Here's the drawing with two shaded views (mm, measured from the low corner). I have some questions. A direction names the side the tool comes from. Give positions to 0.01 mm unless a question says otherwise; leave off trailing zeros. Loops run counter-clockwise (first coordinate to the right, second up) from the corner with the lowest first, then second, coordinate; pieces in that order, holes last. Notation, with made-up numbers: (89.5, 50) - (136.5, 50) arc R12 cw to (136.5, 63) - close; hole circle Ø8 at (86.5, -29). An arc over 180 degrees is marked (long way). Answer as a JSON object with one key per item and string values. Group by question number.
Item 1: Suppose I cut it at B-B on y = 4.5. Write out the boundary of the cut face in (x, z), and give its area (3 significant figures).
Item 2: Will this pin go through, and if not, where does the flat tip stop? pin 1 (4 mm diameter, centred on x = 6.78, y = 6.73, fed in from -Z).
Item 3: Suppose I cut it at A-A on x = 30. Write out the boundary of the cut face in (y, z).
Item 4: Suppose I cut it at C-C on z = 4.75. Count the separate pieces of the cut face and the enclosed holes in it, and give its area (3 significant figures).
Item 5: Please list where these lines run through material, in increasing order: L1, parallel to Y at x = 19, z = 3.25; L2, parallel to Y at x = 30, z = 3.75; L3, parallel to X at y = 10, z = 2.75.
Item 6: Which directions (+Z, -Z, +X, -X, +Y, -Y) give clear straight access to the entire face, cutting with the end or side of a thin tool? Please do the marked faces 4 and 5.
Item 7: Thinking about a two-plate mould opening in X: for the marked faces 1, 2 and 3, which applies, pulls with the +X half, pulls with the -X half, needs draft (parallel to the pull), parting line crosses it, or undercut?
Item 8: Suppose I cut it at D-D on x = 19. Write out the boundary of the cut face in (y, z).
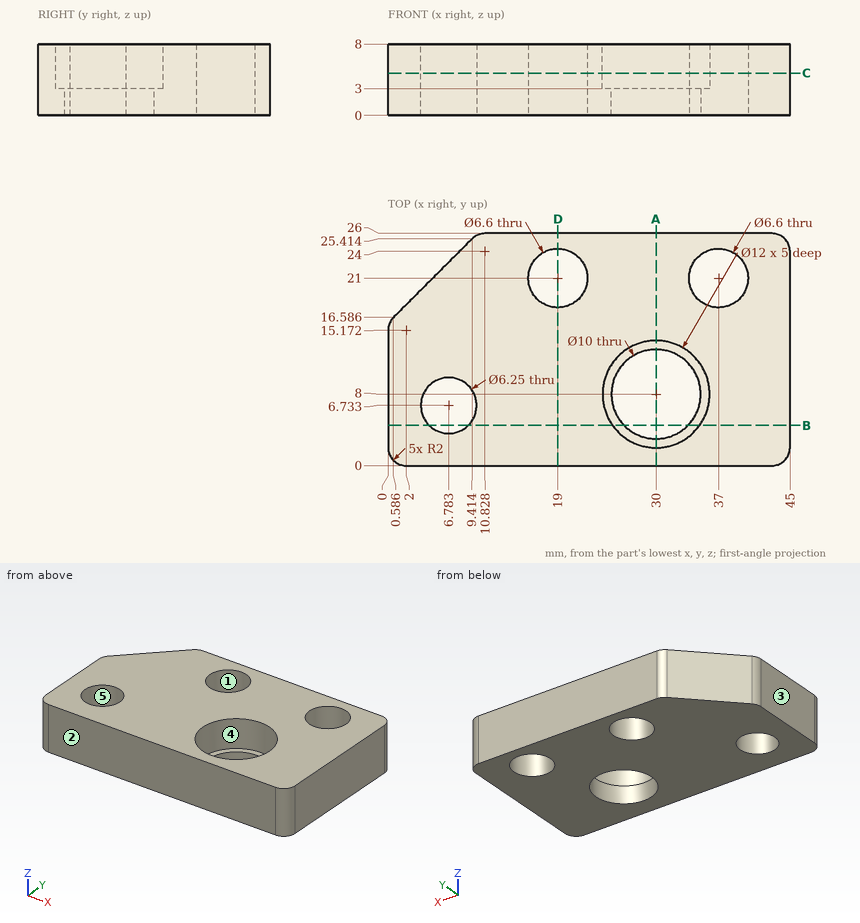
Worked out:
{
 "1": {"outline": "(0, 0) - (4.6, 0) - (4.6, 8) - (0, 8) - close; (8.97, 0) - (26.43, 0) - (26.43, 3) - (25.13, 3) - (25.13, 8) - (8.97, 8) - close; (33.57, 0) - (45, 0) - (45, 8) - (34.87, 8) - (34.87, 3) - (33.57, 3) - close", "area": "255 mm2"},
 "2": {"pin 1": "passes through"},
 "3": {"outline": "(0, 0) - (3, 0) - (3, 3) - (2, 3) - (2, 8) - (0, 8) - close; (13, 0) - (26, 0) - (26, 8) - (14, 8) - (14, 3) - (13, 3) - close"},
 "4": {"separate pieces": "1", "enclosed holes": "4", "area": "905 mm2"},
 "5": {"L1": "y = 0 to 17.7, 24.3 to 26", "L2": "y = 0 to 2, 14 to 26", "L3": "x = 0 to 25.42, 34.58 to 45"},
 "6": {"face 4": "+Z", "face 5": "+Z, -Z"},
 "7": {"face 1": "undercut", "face 2": "needs draft", "face 3": "pulls with the -X half"},
 "8": {"outline": "(0, 0) - (17.7, 0) - (17.7, 8) - (0, 8) - close; (24.3, 0) - (26, 0) - (26, 8) - (24.3, 8) - close"}
}
